Read the model definition and answer for the solid it produces. Units are mm, in the model's axes. Face numbers are marked on the shaded views. A direction names the side the tool comes from. Coordinates: 2 decimals unless noted, no trailing zeros. Write each loop counter-clockwise with the first axis right and the second up, starting at its lowest first coordinate (ties: lowest second). Pieces come first, ordered by that corner, then holes.
(1) Given pin 1 (2.5 mm diameter, centred on x = 10.5, y = 2.5, fed in from +Z); pin 2 (3 mm diameter, centred on x = -52, z = -22, fed in from +Y); pin 3 (8.5 mm diameter, centred on y = 14.5, z = -24.5, fed in from -X); pin 4 (5 mm diameter, centred on x = -26, z = -31.5, fed in from -Y), each flat-ended and moving along its own axis, determine where each tip first touches the part or whether it passes through.
(2) Section D-D on z = -25.5 is taken. Write down the section's boundary in (x, y), then the cut area to 3 significant figures.
(3) Find the intervals of material crossed by probe 1 along X at (y, z) = (2.5, -20); probe 2 along X at (y, z) = (22.75, -20); probe 3 along X at (y, z) = (13, -31), in increasing order.
(4) Section A-A on x = -20 is taken. Write down the section's boundary in (y, z), then the cut area to 3 significant figures.
(5) Section B-B on z = -20 is taken. State how many separate pieces and enclosed holes the cut face has, then the cut area to 3 significant figures.
(6) Which of the six approach directions +Z, -Z, +X, -X, +Y, -Y give full straight-line access (tool end or side, diameter ignored) to the marked faces 5, 6 and 7?
(7) The mould has two halves that part along Z. Classify the marked faces 1, 2, 3 and 4: +Z half, -Z half, draft (parallel to the pull), parting line (faces both ways), or undercut.
(8) Section C-C on y = 25 is taken. Write down the section's boundary in (x, z).
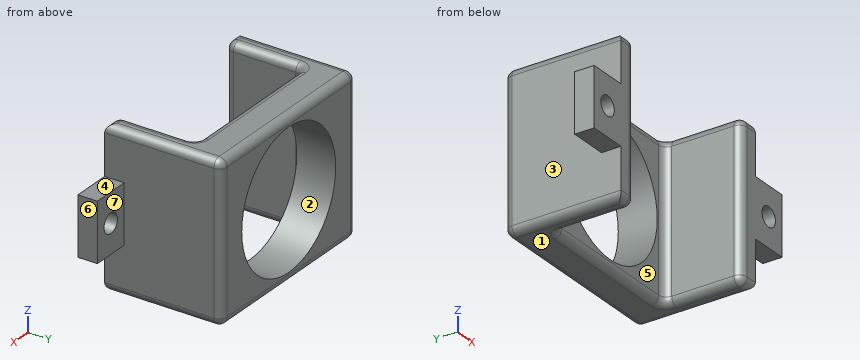
from build123d import *

# Parameters (mm, degrees)
SKETCH1_W             = 5
SKETCH1_H             = 40
BOSS_EXTRUDE1_DEPTH   = 20
BOSS_EXTRUDE1_2_DEPTH = 20
SKETCH2_W             = 50
SKETCH2_H             = 40
SKETCH2_R             = 17.5
BOSS_EXTRUDE2_DEPTH   = 10
SKETCH3_W             = 15
SKETCH3_H             = 15
SKETCH3_R             = 2.5
BOSS_EXTRUDE3_DEPTH   = 5
FILLET1_R             = 2


with BuildPart() as part:
    # Sketch1 → Boss-Extrude1 (new body)
    with BuildSketch(Plane(origin=(0, 0, 0), x_dir=(1, 0, 0), z_dir=(0, 1, 0))):
        with Locations((-42.5, 20)):
            Rectangle(SKETCH1_W, SKETCH1_H)
    extrude(amount=BOSS_EXTRUDE1_DEPTH)



with BuildPart() as body_2:
    # Sketch1 → Boss-Extrude1 2 (new body)
    with BuildSketch(Plane(origin=(0, 0, 0), x_dir=(1, 0, 0), z_dir=(0, 1, 0))):
        with Locations((2.5, 20)):
            Rectangle(SKETCH1_W, SKETCH1_H)
    extrude(amount=BOSS_EXTRUDE1_2_DEPTH)


with BuildPart() as part_1:
    add(part.part)

    add(body_2.part)  # Boss-Extrude2 merges body 2
    # Sketch2 → Boss-Extrude2 (add)
    with BuildSketch(Plane(origin=(0, 20, 0), x_dir=(1, 0, 0), z_dir=(0, 1, 0))):
        with Locations((-20, 20)):
            Rectangle(SKETCH2_W, SKETCH2_H)
        with Locations(Location((-20, 20, 0), (0, 0, 270))):
            Circle(SKETCH2_R, mode=Mode.SUBTRACT)
    extrude(amount=BOSS_EXTRUDE2_DEPTH)

    # Sketch3 → Boss-Extrude3 (add)
    # profile 1 of 2: a face of its own
    with BuildSketch(Plane.XZ):
        with Locations((-47.5, -20)):
            Rectangle(SKETCH3_W, SKETCH3_H)
        with Locations(Location((-50, -20, 0), (0, 0, 270))):
            Circle(SKETCH3_R, mode=Mode.SUBTRACT)
    # profile 2 of 2: a face of its own
    with BuildSketch(Plane.XZ):
        with Locations((7.5, -20)):
            Rectangle(SKETCH3_W, SKETCH3_H)
        with Locations(Location((10, -20, 0), (0, 0, 270))):
            Circle(SKETCH3_R, mode=Mode.SUBTRACT)
    extrude(amount=-BOSS_EXTRUDE3_DEPTH)

    # Fillet1
    fillet1_edges = [part_1.edges().sort_by_distance(p)[0] for p in [
        (-40, 20, -20),
        (-45, 30, -20),
        (-20, 30, 0),
        (5, 30, -20),
        (-20, 30, -40),
        (-20, 20, 0),
        (5, 15, 0),
        (5, 15, -40),
        (-20, 20, -40),
        (0, 0, -20),
        (0, 10, -40),
        (2.5, 0, 0),
        (0, 10, 0),
        (2.5, 0, -40),
        (0, 20, -20),
        (-42.5, 0, -40),
        (-40, 0, -20),
        (-42.5, 0, 0),
        (-45, 15, -40),
        (-40, 10, -40),
        (-40, 10, 0),
        (-45, 15, 0),
    ]]
    fillet(fillet1_edges, radius=FILLET1_R)


solid = part_1.part
Response:
1. pin 1: stops at z = -12.5
1. pin 2: stops at y = 5
1. pin 3: stops at x = -45
1. pin 4: passes through
2. outline: (-55, 0) - (-42, 0) arc R2 ccw to (-40, 2) - (-40, 18) arc R2 cw to (-38, 20) - (-36.61, 20) - (-36.61, 30) - (-43, 30) arc R2 ccw to (-45, 28) - (-45, 5) - (-55, 5) - close; (-3.39, 20) - (-2, 20) arc R2 cw to (0, 18) - (0, 2) arc R2 ccw to (2, 0) - (15, 0) - (15, 5) - (5, 5) - (5, 28) arc R2 ccw to (3, 30) - (-3.39, 30) - close
2. area: 466 mm2
3. probe 1: x = -55 to -52.5, -47.5 to -40, 0 to 7.5, 12.5 to 15
3. probe 2: x = -45 to -37.5, -2.5 to 5
3. probe 3: x = -45 to -40, 0 to 5
4. outline: (20, -38) arc R2 ccw to (22, -40) - (28, -40) arc R2 ccw to (30, -38) - (30, -37.5) - (20, -37.5) - close; (20, -2.5) - (30, -2.5) - (30, -2) arc R2 ccw to (28, 0) - (22, 0) arc R2 ccw to (20, -2) - close
4. area: 46.6 mm2
5. separate pieces: 4
5. enclosed holes: 0
5. area: 398 mm2
6. face 5: +Z, -Z, -Y
6. face 6: +Z, -Z, +X, +Y, -Y
6. face 7: +Z, -Z, +X, +Y
7. face 1: -Z half
7. face 2: undercut
7. face 3: draft
7. face 4: +Z half
8. outline: (-45, -38) arc R2 ccw to (-43, -40) - (3, -40) arc R2 ccw to (5, -38) - (5, -2) arc R2 ccw to (3, 0) - (-43, 0) arc R2 ccw to (-45, -2) - close; hole circle Ø35 at (-20, -20)
